Verification items for the finished model (mm, model axes). A direction names the side the tool comes from. Coordinates: 2 decimals unless noted, no trailing zeros. Write each loop counter-clockwise with the first axis right and the second up, starting at its lowest first coordinate (ties: lowest second). Pieces come first, ordered by that corner, then holes. Notation, with made-up numbers: (80, 50) - (128, 50) arc R28 cw to (128, 70) - close; hole circle Ø7 at (-19, 81.25). An arc over 180 degrees is marked (long way). Answer as CSV lines item,"result". Start each with the question number.
```python
from build123d import *

# Parameters (mm, degrees)
SKETCH1_W                      = 42
SKETCH1_H                      = 42
BOSS_EXTRUDE1_DEPTH            = 60.4
SKETCH2_R                      = 12.5
BOSS_EXTRUDE2_DEPTH            = 2.5
SKETCH4_R                      = 3
BOSS_EXTRUDE3_DEPTH            = 20
CUT_EXTRUDE1_DEPTH             = 47
F_4_2_4_2_DIAMETER_HOLE1_D     = 4.2
CIRPATTERN1_COUNT              = 4
F_3_7_3_7_DIAMETER_HOLE1_D     = 3.7
F_3_7_3_7_DIAMETER_HOLE1_DEPTH = 6
F_3_7_3_7_DIAMETER_HOLE1_TIP   = 1.111592145
FILLET1_R                      = 2
FILLET2_R                      = 1


with BuildPart() as part:
    # Sketch1 → Boss-Extrude1 (new body)
    with BuildSketch(Plane(origin=(0, 0, 0), x_dir=(1, 0, 0), z_dir=(0, 1, 0))):
        Rectangle(SKETCH1_W, SKETCH1_H)
    extrude(amount=-BOSS_EXTRUDE1_DEPTH)

    # Sketch2 → Boss-Extrude2 (add)
    with BuildSketch(Plane(origin=(0, 0, 0), x_dir=(1, 0, 0), z_dir=(0, 1, 0))):
        with Locations(Location((0, 0, 0), (0, 0, 90))):
            Circle(SKETCH2_R)
    extrude(amount=BOSS_EXTRUDE2_DEPTH)

    # Sketch4 → Boss-Extrude3 (add)
    with BuildSketch(Plane(origin=(0, 0, 0), x_dir=(1, 0, 0), z_dir=(0, 1, 0))):
        with Locations(Location((0, 0, 0), (0, 0, 270))):
            Circle(SKETCH4_R)
    extrude(amount=BOSS_EXTRUDE3_DEPTH)

    # Sketch5 → Cut-Extrude1 (cut)
    with BuildSketch(Plane.XZ.offset(60.4)):
        with BuildLine():
            Line((21, 21), (21, 13.75))
            Line((21, 13.75), (17.5, 13.75))
            ThreePointArc((17.5, 13.75), (14.848349571, 14.848349571), (13.75, 17.5))
            Line((13.75, 17.5), (13.75, 21))
            Line((13.75, 21), (21, 21))
        make_face()
    cut_extrude1 = extrude(amount=-CUT_EXTRUDE1_DEPTH, mode=Mode.SUBTRACT)

    # Ø4.2 (4.2) Diameter Hole1 (through all)
    with Locations(Plane(origin=(0, 0, 0), x_dir=(1, 0, 0), z_dir=(0, 1, 0))):
        with Locations((17.5, -17.5)):
            f_4_2_4_2_diameter_hole1 = Hole(F_4_2_4_2_DIAMETER_HOLE1_D / 2)

    # CirPattern1: Cut-Extrude1, Ø4.2 (4.2) Diameter Hole1 ×4 about axis
    cirpattern1_axis = Axis((0, 0, 0), (0, 1, 0))
    add([cut_extrude1.rotate(cirpattern1_axis, i * 360 / CIRPATTERN1_COUNT) for i in range(1, CIRPATTERN1_COUNT)], mode=Mode.SUBTRACT)
    add([f_4_2_4_2_diameter_hole1.rotate(cirpattern1_axis, i * 360 / CIRPATTERN1_COUNT) for i in range(1, CIRPATTERN1_COUNT)], mode=Mode.SUBTRACT)

    # Ø3.7 (3.7) Diameter Hole1
    with Locations(Plane(origin=(0, 0, 0), x_dir=(1, 0, 0), z_dir=(0, 1, 0))):
        with Locations((-5.814342437, 15.974774553), (-16.741731801, -2.95201902), (0, -17), (16.741731801, -2.95201902)):
            Hole(F_3_7_3_7_DIAMETER_HOLE1_D / 2, depth=F_3_7_3_7_DIAMETER_HOLE1_DEPTH)
            with Locations((0, 0, -(F_3_7_3_7_DIAMETER_HOLE1_DEPTH + F_3_7_3_7_DIAMETER_HOLE1_TIP / 2))):  # 118° drill point
                Cone(0, F_3_7_3_7_DIAMETER_HOLE1_D / 2, F_3_7_3_7_DIAMETER_HOLE1_TIP, mode=Mode.SUBTRACT)

    # Fillet1
    fillet1_edges = [part.edges().sort_by_distance(p)[0] for p in [
        (21, -6.7, 21),
        (13.75, -36.9, 21),
        (21, -36.9, 13.75),
        (-21, -6.7, 21),
        (-21, -36.9, 13.75),
        (-13.75, -36.9, 21),
        (21, -6.7, -21),
        (-21, -6.7, -21),
        (-13.75, -36.9, -21),
        (-21, -36.9, -13.75),
        (21, -36.9, -13.75),
        (13.75, -36.9, -21),
    ]]
    fillet(fillet1_edges, radius=FILLET1_R)

    # Fillet2
    fillet2_edges = [part.edges().sort_by_distance(p)[0] for p in [
        (13.75, -60.4, 18.25),
        (-13.75, -60.4, -18.25),
        (0, -60.4, -21),
        (18.25, -60.4, -13.75),
        (21, -60.4, 0),
        (0, -60.4, 21),
        (-18.25, -60.4, 13.75),
        (-21, -60.4, 0),
        (-20.414213562, -60.4, -13.164213562),
        (-20.414213562, -60.4, 13.164213562),
        (-13.164213562, -60.4, -20.414213562),
        (13.164213562, -60.4, -20.414213562),
        (20.414213562, -60.4, -13.164213562),
        (20.414213562, -60.4, 13.164213562),
        (-13.164213562, -60.4, 20.414213562),
        (13.164213562, -60.4, 20.414213562),
        (14.848349571, -60.4, 14.848349571),
        (18.25, -60.4, 13.75),
        (-14.848349571, -60.4, 14.848349571),
        (-13.75, -60.4, 18.25),
        (-14.848349571, -60.4, -14.848349571),
        (-18.25, -60.4, -13.75),
        (14.848349571, -60.4, -14.848349571),
        (13.75, -60.4, -18.25),
    ]]
    fillet(fillet2_edges, radius=FILLET2_R)


solid = part.part
```
1. Cross-section at D-D (z = 6). Record the cut outline in (x, y).
2. Depth check by flat-ended pin: P1, Ø1.2, axis at x = -18, y = -47, coming from the -Z side; P2, Ø3, axis at x = -7.5, z = 13, coming from the +Y side; P3, Ø3, axis at x = 16.74, z = 2.95, coming from the +Y side. Enter the tip coordinate at first touch or a pass-through.
3. Access from +Z, -Z, +X, -X, +Y, -Y to the whole of each face (thin tool, end or side, straight path). Record for faces 5 (the face through (14.9, -36.7, 14.8)), 6 (the face through (-20, -13.4, -18)), 7 (the face through (18, -37, -13.75)).
4. Scan lines: line 1 along Z through (x, y) = (0, -2); line 2 along Z through (x, y) = (17, -4.5); line 3 along Y through (x, z) = (9.5, -6). Record each from-to range of solid material in increasing order. Write a range as from..to.
5. Draft check along X on faces 1 (the face through (18, -37, 13.75)), 2 (the face through (-0.07, -6.92, 17.31)), 3 (the face through (20.4, -6.79, -20.43)), 4 (the face through (15.497, -6.794, 16.869)). Enter one of: pulls with the +X half, pulls with the -X half, needs draft (parallel to the pull), parting line crosses it, or undercut.
6. Cross-section at B-B (y = -41.5). Record the cut outline in (x, z), and give its area (3 significant figures).
7. Cross-section at A-A (z = 0). Record the cut outline in (x, y).
8. Cross-section at C-C (x = -10). Record the cut outline in (y, z).
Completed:
1,outline,"(-21, -59.4) arc R1 ccw to (-20, -60.4) - (20, -60.4) arc R1 ccw to (21, -59.4) - (21, 0) - (10.97, 0) - (10.97, 2.5) - (-10.97, 2.5) - (-10.97, 0) - (-21, 0) - close"
2,P1,"stops at z = -13.75"
2,P2,"stops at y = 0"
2,P3,"stops at y = -6.21"
3,face 5,"+Z, +X, -Y"
3,face 6,"-Z, -X, -Y"
3,face 7,"-Z, +X, -Y"
4,line 1,"z = -21..15.15, 18.85..21"
4,line 2,"z = -21..-19.54, -15.46..1.12, 4.78..15.46, 19.54..21"
4,line 3,"y = -60.4..2.5"
5,face 1,"needs draft"
5,face 2,"undercut"
5,face 3,"pulls with the +X half"
5,face 4,"undercut"
6,outline,"(-21, -11.75) arc R2 ccw to (-19, -13.75) - (-17.5, -13.75) arc R3.75 cw to (-13.75, -17.5) - (-13.75, -19) arc R2 ccw to (-11.75, -21) - (11.75, -21) arc R2 ccw to (13.75, -19) - (13.75, -17.5) arc R3.75 cw to (17.5, -13.75) - (19, -13.75) arc R2 ccw to (21, -11.75) - (21, 11.75) arc R2 ccw to (19, 13.75) - (17.5, 13.75) arc R3.75 cw to (13.75, 17.5) - (13.75, 19) arc R2 ccw to (11.75, 21) - (-11.75, 21) arc R2 ccw to (-13.75, 19) - (-13.75, 17.5) arc R3.75 cw to (-17.5, 13.75) - (-19, 13.75) arc R2 ccw to (-21, 11.75) - close"
6,area,"1,560 mm2"
7,outline,"(-21, -59.4) arc R1 ccw to (-20, -60.4) - (20, -60.4) arc R1 ccw to (21, -59.4) - (21, 0) - (12.5, 0) - (12.5, 2.5) - (3, 2.5) - (3, 20) - (-3, 20) - (-3, 2.5) - (-12.5, 2.5) - (-12.5, 0) - (-21, 0) - close"
8,outline,"(-60.4, -20) arc R1 ccw to (-59.4, -21) - (0, -21) - (0, -7.5) - (2.5, -7.5) - (2.5, 7.5) - (0, 7.5) - (0, 21) - (-59.4, 21) arc R1 ccw to (-60.4, 20) - close"
